Input: part model. Units: mm. Frame: model coordinates. A direction names the side the tool comes from. Give positions to 0.01 mm unless a question says otherwise; leave off trailing zeros. Order: outer loops, then holes, each group sorted by start corner. A loop starts at its lowest first (then second) coordinate and runs counter-clockwise, first axis right, second up. Notation, with made-up numbers: M 43.5,68 L 57.5,68 A21 ccw 57.5,101 Z; hole C 17,83.25 d1. An arc over 180 degrees is marked long. Use a Markdown table: item, result.
Autodesk Inventor part; units mm, degrees
ref_plane "Work Plane1" through (0, 34.7218, 20.3835) normal (0, 0.7071068, 0.7071068) x (-1, 0, 0)
ref_plane "Work Plane2" through (0, 51.2365, 8.0716) normal (0, 0.7071068, 0.7071068) x (1, 0, 0)
ref_plane "Work Plane3" through (0, 31.75, 0) normal (0, -1, 0) x (1, 0, 0)
sketch "Sketch1" plane through (0, 0, 0) normal (0, 1, 0) x (-1, 0, 0)
  circle A0 centre (0, 0) radius 20.3835
  dimension "d0" = 40.767
extrude "Extrusion1" add sketch "Sketch1" along normal blind 34.7218
sketch "Sketch2" plane through (0, 34.7218, 0) normal (0, 1, 0) x (1, 0, 0)
  circle A0 centre (0, 0) radius 20.3835
  line L0 (0, -20.3835) -> (-27.7458, -20.3835)
ref_plane "Work Plane1" through (0, 34.7218, 20.3835) normal (0, 0.7071068, 0.7071068) x (-1, 0, 0)
sketch "Sketch3" plane through (0, 34.7218, 20.3835) normal (0, 0.7071068, 0.7071068) x (-1, 0, 0)
  circle A0 centre (0, -20.3835) radius 20.3835
  circle A1 centre (0, -20.3835) radius 20.3835
  point P0 (0, 10.1387)
extrude "Extrusion2" add sketch "Sketch3" along normal blind 34.7218
sketch "Sketch4" plane through (0, 0, 0) normal (0, -1, 0) x (1, 0, 0)
  circle A0 centre (0, 0) radius 16.7767
  dimension "d6" = 33.5534
extrude "Extrusion3" cut sketch "Sketch4" against normal blind 31.75
sketch "Sketch5" plane through (0, 73.6871, 30.5222) normal (0, 0.7071068, 0.7071068) x (1, 0, 0)
  circle A0 centre (0, 0) radius 16.7767
  point P0 (0, -30.5222)
  dimension "d9" = 33.5534
extrude "Extrusion4" cut sketch "Sketch5" against normal blind 31.75
ref_plane "Work Plane2" through (0, 51.2365, 8.0716) normal (0, 0.7071068, 0.7071068) x (1, 0, 0)
ref_plane "Work Plane3" through (0, 31.75, 0) normal (0, -1, 0) x (1, 0, 0)
revolve "Revolution1" add sketch "Sketch2" angle 45 about axis through (0, 34.7218, 20.3835) along (1, 0, 0)
ref_plane "Work Plane4" through (0, 34.7218, 20.3835) normal (-1, 0, 0) x (0, -1, 0)
sketch "Sketch6" plane through (0, 34.7218, 20.3835) normal (-1, 0, 0) x (0, -1, 0)
  line L0 (0, 33.7996) -> (-51.2396, 33.7996)
  point P0 (34.7218, -20.3835)
ref_plane "Work Plane5" through (0, 34.7218, 54.1831) normal (-0.7071068, 0, -0.7071068) x (0, 1, 0)
sketch "Sketch8" plane through (0, 34.7218, 20.3835) normal (-1, 0, 0) x (0, -1, 0)
  line L0 (-28.3776, -24.1748) -> (-4.6518, -0.449)
  line L1 (2.9718, -3.6068) -> (2.9718, -37.1602)
  line L2 (-4.6518, -0.449) -> (2.9718, -3.6068)
  point P0 (34.7218, -20.3835)
sketch "Sketch9" plane through (0, 31.75, 0) normal (0, -1, 0) x (1, 0, 0)
  circle A0 centre (0, 0) radius 12.7
  dimension "d17" = 25.4
extrude "Extrusion5" cut sketch "Sketch9" against normal blind 2.9718
sketch "Sketch10" plane through (0, 51.2365, 8.0716) normal (0, 0.7071068, 0.7071068) x (1, 0, 0)
  circle A0 centre (0, 0) radius 12.7
  point P0 (0, -30.5222)
  dimension "d20" = 25.4
extrude "Extrusion6" cut sketch "Sketch10" against normal blind 2.9718
sketch "Sketch11" plane through (0, 34.7218, 0) normal (0, -1, 0) x (1, 0, 0)
  circle A0 centre (0, 0) radius 12.7
  line L0 (28.5369, 20.3835) -> (-28.5369, 20.3835)
revolve "Revolution2" cut sketch "Sketch11" angle 45 about axis through (0, 34.7218, 20.3835) along (1, 0, 0)
properties part number "45 Elbow 1 Inch"
1) Mould query, pull axis Z, two halves, no side actions, for faces 3 (the face through (16.7, 75.76, 28.45)), 4 (the face through (16, 15.65, 5.04)), 5 (the face through (17, 0, -3)). Classes: released by +Z, released by -Z, zero draft, split by the parting line, or undercut.
Response values:
| item | result |
|---|---|
| face 3 | released by +Z |
| face 4 | undercut |
| face 5 | zero draft |
2) Material intervals for line 1 (Z direction, x = 0, y = 32.65); line 2 (Z direction, x = 0, y = 24); line 3 (Y direction, x = 13.5, z = 22.5), sorted ascending. Write a range as from..to.
Response values:
| item | result |
|---|---|
| line 1 | z = -20.38..-12.7, 12.7..20.38 |
| line 2 | z = -20.38..-16.78, 16.78..20.38 |
| line 3 | y = 44.07..51.58, 79.75..81.71 |
3) Reachability of faces 1 (the face through (-12.505, 53.927, 5.379)), 2 (the face through (-3, 31.75, 13)) from +Z, -Z, +X, -X, +Y, -Y: full face, straight path, thin tool, end or side. Return the list, or none.
Response values:
| item | result |
|---|---|
| face 1 | none |
| face 2 | -Y |
4) Cut plane A-A on y = 9. Return loops of the section in (x, z).
Response values:
| item | result |
|---|---|
| outline | C 0,0 d40.77; hole C 0,0 d33.55 |
5) First-contact query: pin 1 Ø1.5 at (y, z) = (64, 7.5) entering from +X; pin 2 Ø6 at (x, z) = (4, 27) entering from +Y; pin 3 Ø1.5 at (x, z) = (15, 36.5) entering from -Y. Flat tips, straight axial feed; report the tip coordinate or a pass-through.
Response values:
| item | result |
|---|---|
| pin 1 | stops at x = 18.44 |
| pin 2 | stops at y = 50.36 |
| pin 3 | stops at y = 58.81 |
